Could you check a few things on this drawing? It's one solid part, dimensions in mm from its lowest x, y, z. A direction names the side the tool comes from. Round coordinates to 2 decimals unless told otherwise and drop trailing zeros. Loops run counter-clockwise (first coordinate to the right, second up) from the corner with the lowest first, then second, coordinate; pieces in that order, holes last. Notation, with made-up numbers: M 0.5,-22 L 13.5,-22 A13 ccw 13.5,-14 Z; hole C 11.25,81.5 d8. An arc over 180 degrees is marked long. Answer as a JSON object with one key per item and string values.
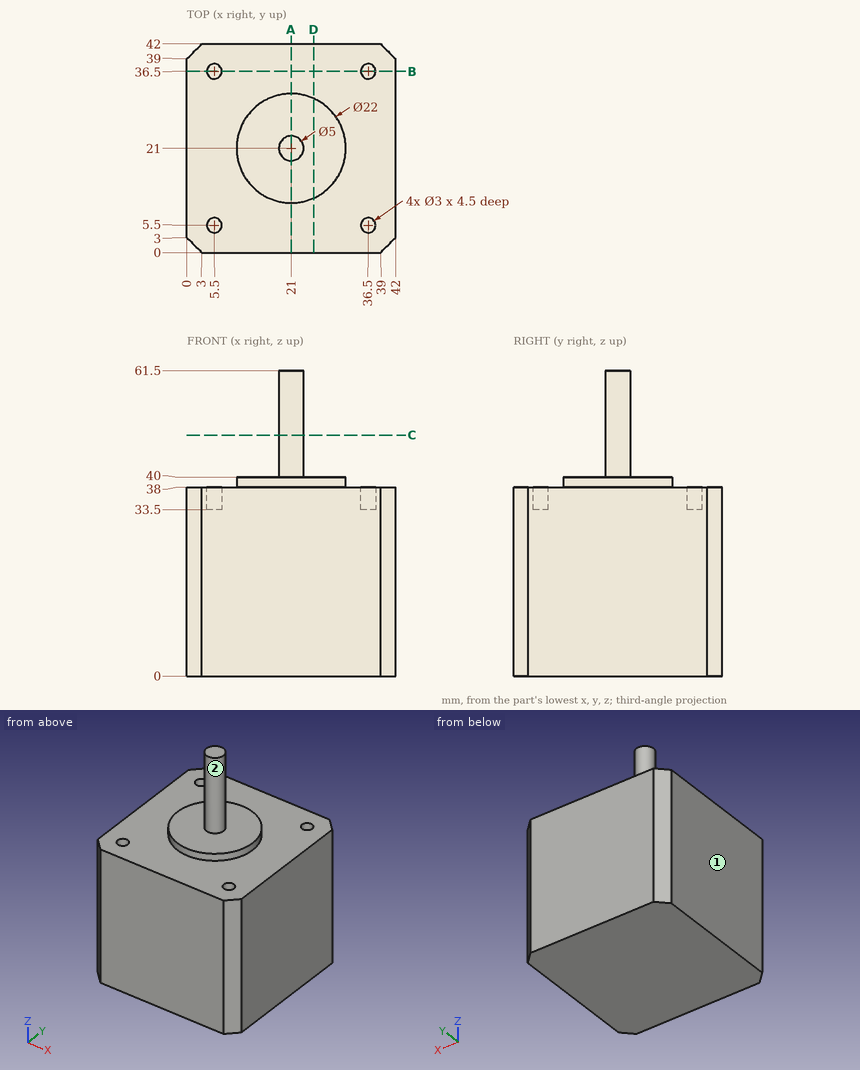
Item 1: I want a section at B-B, the plane y = 36.5. Please give me the cut outline in (x, z).
Resolved:
{"outline": "M 0,0 L 42,0 L 42,38 L 38,38 L 38,33.5 L 35,33.5 L 35,38 L 7,38 L 7,33.5 L 4,33.5 L 4,38 L 0,38 Z"}
Item 2: I want a section at D-D, the plane x = 25.5. Please give me the cut outline in (y, z).
Resolved:
{"outline": "M 0,0 L 42,0 L 42,38 L 31.04,38 L 31.04,40 L 10.96,40 L 10.96,38 L 0,38 Z"}
Item 3: Please list where these lines run through material, in increasing order: probe 1 along Y at (x, z) = (36.5, 36); probe 2 along X at (y, z) = (5, 36). Write a range as from..to.
Resolved:
{"probe 1": "0..4, 7..35, 38..42", "probe 2": "0..4.09, 6.91..35.09, 37.91..42"}
Item 4: On a 3-axis mill with a long thin cutter (end or side, diameter ignored), from which of +Z, -Z, +X, -X, +Y, -Y can I reach the whole of each face in a straight line? I mean the marked faces 1 and 2. Say none if no direction works.
Resolved:
{"face 1": "+Z, -Z, -X, +Y, -Y", "face 2": "+Z"}
Item 5: I want a section at C-C, the plane z = 48.5. Please give me the cut outline in (x, y), then the cut area to 3 significant figures.
Resolved:
{"outline": "C 21,21 d5", "area": "19.6 mm²"}
Item 6: I want a section at A-A, the plane x = 21. Please give me the cut outline in (y, z), then the cut area to 3 significant figures.
Resolved:
{"outline": "M 0,0 L 42,0 L 42,38 L 32,38 L 32,40 L 23.5,40 L 23.5,61.5 L 18.5,61.5 L 18.5,40 L 10,40 L 10,38 L 0,38 Z", "area": "1,750 mm²"}
Item 7: I'm going to push flat-ended pins straight in: pin 1 Ø3.5 at (x, y) = (36, 6) entering from +Z; pin 2 Ø0.9 at (x, y) = (6, 5.5) entering from +Z. Where does each tip first touch, or does it pass through?
Resolved:
{"pin 1": "z = 38", "pin 2": "z = 33.5"}
